from build123d import *

# Parameters (mm, degrees)
SKETCH6_W               = 17
SKETCH6_H               = 1
SKETCH6_W_2             = 66.3
SKETCH6_H_2             = 49
FILM_PLANE_DEPTH        = 3
CUT_EXTRUDE2_DEPTH      = 1.3
NOTCH_W                 = 6.8
NOTCH_H                 = 2.5
NOTCH_CUT_DEPTH         = 4.1
SKETCH10_W              = 6.297854397
SKETCH10_H              = 3.8
CUT_EXTRUDE4_DEPTH      = 0.5
CUT_EXTRUDE5_DEPTH      = 1.5
CUT_EXTRUDE6_DEPTH      = 111.449366381
CUT_EXTRUDE6_DEPTH_BACK = 5
SKETCH_1_W              = 1.5
SKETCH_1_H              = 55
OUTLET_DEPTH            = 2
SKETCH_6_W              = 1.5
SKETCH_6_H              = 2
EXTRUDE_1_DEPTH         = 20


with BuildPart() as part:
    # Sketch3 → body section 0
    with BuildSketch(Plane(origin=(0, 0, 0), x_dir=(0, 0, -1), z_dir=(1, 0, 0))):
        with BuildLine():
            Line((0, 61), (16, 61.75))
            Line((16, 61.75), (16, 3.25))
            Line((16, 3.25), (0, 4))
            Line((0, 4), (0, 61))
        make_face()
    # Sketch2 → body section 1
    with BuildSketch(Plane(origin=(92, 0, 0), x_dir=(0, 0, -1), z_dir=(1, 0, 0))):
        with BuildLine():
            Line((0, 61), (20, 61.75))
            Line((20, 61.75), (20, 3.25))
            Line((20, 3.25), (0, 4))
            Line((0, 4), (0, 61))
        make_face()
    loft()

    # Sketch6 → film plane (cut)
    with BuildSketch(Plane.XY):
        with Locations((15.3, 57.7)):
            Rectangle(SKETCH6_W, SKETCH6_H)
        with Locations((39.95, 32.7)):
            Rectangle(SKETCH6_W_2, SKETCH6_H_2)
    extrude(amount=-FILM_PLANE_DEPTH, mode=Mode.SUBTRACT)

    # Sketch7 → Cut-Extrude2 (cut)
    with BuildSketch(Plane.XY):
        Polygon((77.5, 5.25), (77.5, 59.75), (0, 59.75), (0, 4), (2.4, 4), (2.4, 5.25), align=None)
        Polygon((23.8, 58.2), (23.8, 57.2), (73.1, 57.2), (73.1, 8.2), (6.8, 8.2), (6.8, 58.2), align=None, mode=Mode.SUBTRACT)
    extrude(amount=-CUT_EXTRUDE2_DEPTH, mode=Mode.SUBTRACT)

    # notch → notch-cut (cut)
    with BuildSketch(Plane.XY.offset(-1.3)):
        with Locations((3.4, 56.95)):
            Rectangle(NOTCH_W, NOTCH_H)
    extrude(amount=-NOTCH_CUT_DEPTH, mode=Mode.SUBTRACT)

    # Sketch10 → Cut-Extrude4 (cut)
    with BuildSketch(Plane(origin=(-0.694339623, 0, -15.969811321), x_dir=(-0.9990561583550596, 0, 0.04343722427630701), z_dir=(-0.043437224276307015, 0, -0.9990561583550597))):
        with Locations((-89.632983856, 49.35)):
            Rectangle(SKETCH10_W, SKETCH10_H)
    extrude(amount=-CUT_EXTRUDE4_DEPTH, mode=Mode.SUBTRACT)

    # Sketch11 → Cut-Extrude5 (cut)
    with BuildSketch(Plane(origin=(-0.694339623, 0, -15.969811321), x_dir=(-0.9990561583550596, 0, 0.04343722427630701), z_dir=(-0.043437224276307015, 0, -0.9990561583550597))):
        with BuildLine():
            Line((-72.5, 14.5), (-64, 14.5))
            ThreePointArc((-64, 14.5), (-62.232233047, 15.232233047), (-61.5, 17))
            Line((-61.5, 17), (-61.5, 48))
            ThreePointArc((-61.5, 48), (-62.232233047, 49.767766953), (-64, 50.5))
            Line((-64, 50.5), (-72.5, 50.5))
            ThreePointArc((-72.5, 50.5), (-74.267766953, 49.767766953), (-75, 48))
            Line((-75, 48), (-75, 17))
            ThreePointArc((-75, 17), (-74.267766953, 15.232233047), (-72.5, 14.5))
        make_face()
        with BuildLine():
            Line((-24.5, 14.5), (-16, 14.5))
            ThreePointArc((-16, 14.5), (-14.232233047, 15.232233047), (-13.5, 17))
            Line((-13.5, 17), (-13.5, 48))
            ThreePointArc((-13.5, 48), (-14.232233047, 49.767766953), (-16, 50.5))
            Line((-16, 50.5), (-24.5, 50.5))
            ThreePointArc((-24.5, 50.5), (-26.267766953, 49.767766953), (-27, 48))
            Line((-27, 48), (-27, 17))
            ThreePointArc((-27, 17), (-26.267766953, 15.232233047), (-24.5, 14.5))
        make_face()
    extrude(amount=-CUT_EXTRUDE5_DEPTH, mode=Mode.SUBTRACT)

    # Sketch5 → Cut-Extrude6 (cut, two sides: drawn at the far end of the back side and taken through both)
    with BuildSketch(Plane(origin=(0, 61, 0), x_dir=(1, 0, 0), z_dir=(0, 1, 0)).offset(-CUT_EXTRUDE6_DEPTH_BACK)):
        Polygon((0, 1.5), (18, 1.5), (20, 0), (0, 0), align=None)
    extrude(amount=CUT_EXTRUDE6_DEPTH + CUT_EXTRUDE6_DEPTH_BACK, mode=Mode.SUBTRACT)

    # 草图1 → outlet (cut)
    with BuildSketch(Plane(origin=(92, 0, 0), x_dir=(0, 0, -1), z_dir=(1, 0, 0))):
        with Locations((3, 32.5)):
            Rectangle(SKETCH_1_W, SKETCH_1_H)
    extrude(amount=-OUTLET_DEPTH, mode=Mode.SUBTRACT)

    # 草图6 → 凸台-拉伸1 (add)
    with BuildSketch(Plane.XY):
        with Locations((91.25, 62)):
            Rectangle(SKETCH_6_W, SKETCH_6_H)
        with Locations((91.25, 3)):
            Rectangle(SKETCH_6_W, SKETCH_6_H)
    extrude(amount=-EXTRUDE_1_DEPTH)


solid = part.part
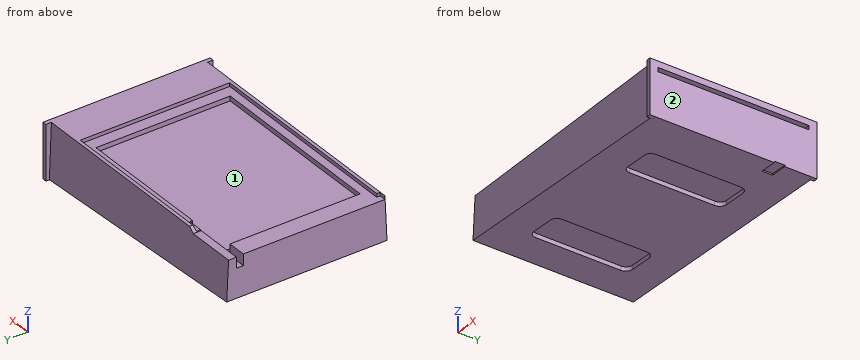
For this review, take the finished solid that the model builds, in its own axes (mm). Face numbers are marked on the shaded views. Give positions to 0.01 mm unless a question says otherwise; leave off trailing zeros. Loops run counter-clockwise (first coordinate to the right, second up) from the corner with the lowest first, then second, coordinate; pieces in that order, holes last.
Item 1: For line 1 along X through (y, z) = (53, -1.75); line 2 along Z through (x, y) = (26.5, 26); line 3 along Z through (x, y) = (72, 48), list the stretches that pass through material, from the lowest coordinate up.
Item 2: Draft analysis for pull direction Y (two halves, no side actions). For the marked faces 1 and 2, state which applies: +Y half, -Y half, draft (parallel to the pull), parting line (faces both ways), or undercut.
Item 3: Take a section at A-A, the plane y = 13. State the section outline as (x, z) points, and give its area (3 significant figures).
Item 4: Insertion check: pin 1 (1 mm diameter, centred on x = 27.5, z = -1, fed in from +Y); pin 2 (4 mm diameter, centred on x = 56, y = 14.5, fed in from -Z); pin 3 (1.4 mm diameter, centred on x = 1, z = -0.5, fed in from +Y). Each pin has a flat end and moves straight along its axis. Give the tip position at first contact, or say it passes through.
Item 5: Take a section at B-B, the plane y = 22. State the section outline as (x, z) points, and give its area (3 significant figures).
Calculated:
1. line 1: x = 0 to 6.8, 73.1 to 92
1. line 2: z = -17.15 to -3
1. line 3: z = -17.63 to -3
2. face 1: undercut
2. face 2: draft
3. outline: (0, -16) - (92, -20) - (92, -3.75) - (90, -3.75) - (90, -2.25) - (92, -2.25) - (92, 0) - (77.5, 0) - (77.5, -1.3) - (73.1, -1.3) - (73.1, -3) - (6.8, -3) - (6.8, -1.3) - (0, -1.3) - close
3. area: 1,440 mm2
4. pin 1: stops at y = 61.07
4. pin 2: stops at z = -18.52
4. pin 3: stops at y = 4
5. outline: (0, -16) - (12.79, -16.56) - (12.86, -15.06) - (26.35, -15.64) - (26.28, -17.14) - (60.75, -18.64) - (60.81, -17.14) - (74.3, -17.73) - (74.23, -19.23) - (92, -20) - (92, -3.75) - (90, -3.75) - (90, -2.25) - (92, -2.25) - (92, 0) - (77.5, 0) - (77.5, -1.3) - (73.1, -1.3) - (73.1, -3) - (6.8, -3) - (6.8, -1.3) - (0, -1.3) - close
5. area: 1,400 mm2
